```python
from build123d import *

# Parameters (mm, degrees)
EXTRUDE_1_DEPTH     = 14
SKETCH_2_R          = 2.75
CUT_EXTRUDE_1_DEPTH = 34.481338086


with BuildPart() as part:
    # 草图1 → 凸台-拉伸1 (new body)
    with BuildSketch(Plane.XY):
        with BuildLine():
            Line((-1, 0), (-9, 0))
            Line((-9, 0), (-9, -22))
            Line((-9, -22), (-21, -22))
            Line((-21, -22), (-21, -28))
            Line((-21, -28), (21, -28))
            Line((21, -28), (21, -22))
            Line((21, -22), (9, -22))
            Line((9, -22), (9, 0))
            Line((9, 0), (1, 0))
            Line((1, 0), (1, -10.171572875))
            ThreePointArc((1, -10.171572875), (0, -16), (-1, -10.171572875))
            Line((-1, -10.171572875), (-1, 0))
        make_face()
    extrude(amount=EXTRUDE_1_DEPTH)

    # 草图2 → 切除-拉伸1 (cut, through all)
    with BuildSketch(Plane(origin=(0, -22, 0), x_dir=(1, 0, 0), z_dir=(0, 1, 0))):
        with Locations(Location((-16, -7, 0), (0, 0, 180))):
            Circle(SKETCH_2_R)
        with Locations(Location((16, -7, 0), (0, 0, 180))):
            Circle(SKETCH_2_R)
    extrude(amount=-CUT_EXTRUDE_1_DEPTH, mode=Mode.SUBTRACT)


solid = part.part
```
Check sheet for the modelled part. Datum: model origin and axes. Units: mm. A direction names the side the tool comes from. Coordinates: 2 decimals unless noted, no trailing zeros. Order: outer loops, then holes, each group sorted by start corner. A loop starts at its lowest first (then second) coordinate and runs counter-clockwise, first axis right, second up. Notation, with made-up numbers: (76.25, -39) -> (98.25, -39) arc R9 cw to (98.25, -23) -> close; hole circle Ø6 at (55, 66.5). An arc over 180 degrees is marked (long way). Write item = value, one per line. Start each with the question number.
1) Cross-section at D-D (y = -13). Enter the section's corners in (x, z), then the cut area to 3 significant figures.
2) Access from +Z, -Z, +X, -X, +Y, -Y to the whole of each face (thin tool, end or side, straight path). Record for faces 1 (the flat face through (-9, -11, 7)), 2 (the flat face through (-21, -25, 7)), 3 (the flat face through (-1, -5, 7)), 4 (the flat face through (12, -22, 7)).
3) Go/stop test with flat-tipped pins: P1, Ø3.5, axis at x = 0, y = -13, coming from the -Z side; P2, Ø7, axis at y = -9.5, z = 4.5, coming from the -X side; P3, Ø7, axis at x = 16, z = 7, coming from the +Y side; P4, Ø5, axis at y = -3.5, z = 8.5, coming from the +X side. Record where each tip stops, or that it passes through.
4) Cross-section at B-B (x = -16). Enter the section's corners in (y, z).
5) Cross-section at A-A (z = 7). Enter the section's corners in (x, y).
6) Material ranges on L1, parallel to Z at x = -16, y = -23.2; L2, parallel to X at y = -6, z = 8; L3, parallel to Y at x = 0, z = 3.5, recorded low to high.
7) Mould release check, pull along X, two halves, no side actions. Record for faces 5 (the cylindrical face through (0, -16, 7)), 6 (the flat face through (-13.6, -22, 5.3)), 7 (the cylindrical face through (-13.253, -24.958, 7.121)), 8 (the flat face through (21, -25, 7)): +X half, -X half, draft (parallel to the pull), parting line (faces both ways), or undercut.
8) Cross-section at C-C (y = -24.25). Enter the section's corners in (x, z).
Ans:
q1.outline = (-9, 0) -> (-3, 0) -> (-3, 14) -> (-9, 14) -> close; (3, 0) -> (9, 0) -> (9, 14) -> (3, 14) -> close
q1.area = 168 mm²
q2.face_1 = +Z, -Z, -X, +Y
q2.face_2 = +Z, -Z, -X, +Y, -Y
q2.face_3 = +Z, -Z, +Y
q2.face_4 = +Z, -Z, +X, +Y
q3.P1 = through
q3.P2 = -9
q3.P3 = -22
q3.P4 = 9
q4.outline = (-28, 0) -> (-22, 0) -> (-22, 4.25) -> (-28, 4.25) -> close; (-28, 9.75) -> (-22, 9.75) -> (-22, 14) -> (-28, 14) -> close
q5.outline = (-21, -28) -> (-18.75, -28) -> (-18.75, -22) -> (-21, -22) -> close; (-13.25, -28) -> (13.25, -28) -> (13.25, -22) -> (9, -22) -> (9, 0) -> (1, 0) -> (1, -10.17) arc R3 cw (long way) to (-1, -10.17) -> (-1, 0) -> (-9, 0) -> (-9, -22) -> (-13.25, -22) -> close; (18.75, -28) -> (21, -28) -> (21, -22) -> (18.75, -22) -> close
q6.L1 = 0 to 4.25, 9.75 to 14
q6.L2 = -9 to -1, 1 to 9
q6.L3 = -28 to -16
q7.face_5 = undercut
q7.face_6 = draft
q7.face_7 = undercut
q7.face_8 = +X half
q8.outline = (-21, 0) -> (21, 0) -> (21, 14) -> (-21, 14) -> close; hole circle Ø5.5 at (-16, 7); hole circle Ø5.5 at (16, 7)
